```python
from build123d import *

# Parameters (mm, degrees)
SKETCH1_W                  = 25
SKETCH1_H                  = 14
F_6_0MM_DOWEL_HOLE1_D      = 6
CIRPATTERN1_COUNT          = 4
F_4_0MM_DOWEL_HOLE1_REACH  = 63.636
F_4_0MM_DOWEL_HOLE1_BORE_R = 2


with BuildPart() as part:
    # Sketch1 → Revolve2 (revolve)
    with BuildSketch(Plane(origin=(0, 0, 0), x_dir=(1, 0, 0), z_dir=(0, 1, 0)), mode=Mode.PRIVATE) as revolve2_sk:
        with Locations((0, 18)):
            Rectangle(SKETCH1_W, SKETCH1_H)
    revolve(revolve2_sk.sketch.rotate(Axis((-25.731009954, 0, 0), (1, 0, 0)), 180), axis=Axis((-25.731009954, 0, 0), (1, 0, 0)))

    # Ø6.0mm Dowel Hole1 (through all)
    with Locations(Plane(origin=(12.5, 0, 0), x_dir=(0, 0, -1), z_dir=(1, 0, 0))):
        with Locations((0, 17)):
            f_6_0mm_dowel_hole1 = Hole(F_6_0MM_DOWEL_HOLE1_D / 2)

    # CirPattern1: Ø6.0mm Dowel Hole1 ×4 about axis
    cirpattern1_axis = Axis((0, 0, 0), (1, 0, 0))
    for i in range(1, CIRPATTERN1_COUNT):
        add(f_6_0mm_dowel_hole1.rotate(cirpattern1_axis, i * 360 / CIRPATTERN1_COUNT), mode=Mode.SUBTRACT)

    # Ø4.0mm Dowel Hole1 bore (on position points) → Ø4.0mm Dowel Hole1 (cut, up to next)
    with BuildSketch(Plane(origin=(0, -17.677561289, -17.67777777), x_dir=(0, -0.7071111108, 0.707102451547), z_dir=(0, -0.707102451547, -0.7071111108)), mode=Mode.PRIVATE) as f_4_0mm_dowel_hole1_sk1:
        Circle(F_4_0MM_DOWEL_HOLE1_BORE_R)
    f_4_0mm_dowel_hole1_tool1 = extrude(f_4_0mm_dowel_hole1_sk1.sketch, amount=-F_4_0MM_DOWEL_HOLE1_REACH, mode=Mode.PRIVATE) & part.part
    add(f_4_0mm_dowel_hole1_tool1.solids().sort_by_distance((0, -17.677561, -17.677778))[0], mode=Mode.SUBTRACT)


solid = part.part
```
Verification items for the finished model (mm, model axes). Coordinates: 2 decimals unless noted, no trailing zeros. Loops run counter-clockwise (first coordinate to the right, second up) from the corner with the lowest first, then second, coordinate; pieces in that order, holes last. Notation, with made-up numbers: (-4, 65) -> (5, 65) arc R16 cw to (5, 86) -> close; hole circle Ø3 at (87.5, 15.25). An arc over 180 degrees is marked (long way). Answer in a Markdown table with one row per item.
1) Draft check along Z on faces 1 (the face through (0.18, 9.58, 23.09)), 2 (the face through (-12.5, 11, -5)), 3 (the face through (-0.17, 0.65, 14.07)). Enter one of: released by +Z, released by -Z, zero draft, split by the parting line, or undercut.
The answers:
| item | result |
|---|---|
| face 1 | split by the parting line |
| face 2 | zero draft |
| face 3 | undercut |
2) Section check B-B (x = 10). Record the cut outline in (y, z), and give its area (3 significant figures).
The answers:
| item | result |
|---|---|
| outline | circle Ø50 at (0, 0); hole circle Ø6 at (-17, 0); hole circle Ø22 at (0, 0); hole circle Ø6 at (0, -17); hole circle Ø6 at (0, 17); hole circle Ø6 at (17, 0) |
| area | 1,470 mm2 |
3) Section check A-A (z = 0). Record the cut outline in (x, y), and give its area (3 significant figures).
The answers:
| item | result |
|---|---|
| outline | (-12.5, -25) -> (12.5, -25) -> (12.5, -20) -> (-12.5, -20) -> close; (-12.5, -14) -> (12.5, -14) -> (12.5, -11) -> (-12.5, -11) -> close; (-12.5, 11) -> (12.5, 11) -> (12.5, 14) -> (-12.5, 14) -> close; (-12.5, 20) -> (12.5, 20) -> (12.5, 25) -> (-12.5, 25) -> close |
| area | 400 mm2 |
4) Depth check by flat-ended pin: P1, Ø8, axis at y = 0, z = -17, coming from the -X side; P2, Ø4, axis at x = -1.5, y = -9.5, coming from the +Z side; P3, Ø4, axis at x = 10, z = 19, coming from the -Y side; P4, Ø10, axis at x = 5, y = 7.5, coming from the +Z side. Enter the tip coordinate at first touch or a pass-through.
The answers:
| item | result |
|---|---|
| P1 | stops at x = -12.5 |
| P2 | stops at z = 23.85 |
| P3 | stops at y = -18.33 |
| P4 | stops at z = 24.87 |
5) Scan lines: line 1 along Y through (x, z) = (4, 0); line 2 along Y through (x, z) = (1.25, -15.5); line 3 along Z through (x, y) = (3.5, -10). Record each from-to range of solid material in increasing order. Write a range as from..to.
The answers:
| item | result |
|---|---|
| line 1 | y = -25..-20, -14..-11, 11..14, 20..25 |
| line 2 | y = -19.62..-17.71, -13.29..-2.6, 2.6..19.62 |
| line 3 | z = -22.91..-4.58, 4.58..22.91 |
6) Section check C-C (y = 17). Record the cut outline in (x, z).
The answers:
| item | result |
|---|---|
| outline | (-12.5, -18.33) -> (12.5, -18.33) -> (12.5, -3) -> (-12.5, -3) -> close; (-12.5, 3) -> (12.5, 3) -> (12.5, 18.33) -> (-12.5, 18.33) -> close |
